from build123d import *

# Parameters (mm, degrees)
ESQUISSE1_R             = 4.415
BOSS_EXTRU_1_DEPTH      = 14.46
ESQUISSE4_R             = 2.9
ENL_V_MAT_EXTRU_1_DEPTH = 14.46
ESQUISSE6_R             = 3.415
ENL_V_MAT_EXTRU_2_DEPTH = 7


with BuildPart() as part:
    # Esquisse1 → Boss.-Extru.1 (new body)
    with BuildSketch(Plane.XY):
        Circle(ESQUISSE1_R)
    extrude(amount=BOSS_EXTRU_1_DEPTH)

    # Esquisse4 → Enlèv. mat.-Extru.1 (cut)
    with BuildSketch(Plane.XY.offset(14.46)):
        Circle(ESQUISSE4_R)
    extrude(amount=-ENL_V_MAT_EXTRU_1_DEPTH, mode=Mode.SUBTRACT)

    # Esquisse6 → Enlèv. mat.-Extru.2 (cut)
    with BuildSketch(Plane.XY.offset(14.46)):
        Circle(ESQUISSE6_R)
    extrude(amount=-ENL_V_MAT_EXTRU_2_DEPTH, mode=Mode.SUBTRACT)


solid = part.part
Could you check a few things on this model? Use its own coordinates, in mm. A direction names the side the tool comes from. Give positions to 0.01 mm unless a question says otherwise; leave off trailing zeros. Order: outer loops, then holes, each group sorted by start corner. A loop starts at its lowest first (then second) coordinate and runs counter-clockwise, first axis right, second up. Notation, with made-up numbers: (49, -37) - (54, -37) arc R18 ccw to (54, -13) - close; hole circle Ø3 at (-3.5, -2.5). An arc over 180 degrees is marked (long way). One line per question, with ' | ' between items. Start each with the question number.
Item 1: I need wall thicknesses on probe 1 along Y at (x, z) = (0, 9.25) (3 decimals); probe 2 along Y at (x, z) = (0, 5.5) (3 decimals); probe 3 along Z at (x, y) = (0.75, 3.25). Which ranges of each line are inside material? Lowest first, please. Write a range as [from, to].
Item 2: I want a section at C-C on z = 3. Write out the boundary of the cut face in (x, y) (3 decimals), then the cut area to 3 significant figures.
Item 3: I want a section at B-B on y = 1. Write out the boundary of the cut face in (x, z), then the cut area to 3 significant figures.
Item 4: I want a section at A-A on x = 0. Write out the boundary of the cut face in (y, z) (3 decimals).
Item 5: I'm going to push a flat-ended pin straight in: pin 1 Ø5 at (x, z) = (-3, 2) entering from +Y. Where does the tip first touch, or does it pass through?
Item 6: For faces 4 (the cylindrical face through (-0.445, 3.386, 11.009)), 5 (the flat face through (2, -3, 14.46)), which set-ups out of +Z, -Z, +X, -X, +Y, -Y let a thin tool reach every point of the face, with its end or its side?
Item 7: Thinking about a two-plate mould opening in X: for faces 1 (the cylindrical face through (-2.9, 0.1, 3.8)), 2 (the flat face through (1, -3, 0)), 3 (the cylindrical face through (-1, -4.3, 7.1)), which applies, pulls with the +X half, pulls with the -X half, needs draft (parallel to the pull), parting line crosses it, or undercut?
Verdict:
1) probe 1: [-4.415, -3.415], [3.415, 4.415] | probe 2: [-4.415, -2.9], [2.9, 4.415] | probe 3: [0, 7.46]
2) outline: circle Ø8.83 at (0, 0); hole circle Ø5.8 at (0, 0) | area: 34.8 mm^2
3) outline: (-4.3, 0) - (-2.72, 0) - (-2.72, 7.46) - (-3.27, 7.46) - (-3.27, 14.46) - (-4.3, 14.46) - close; (2.72, 0) - (4.3, 0) - (4.3, 14.46) - (3.27, 14.46) - (3.27, 7.46) - (2.72, 7.46) - close | area: 38.0 mm^2
4) outline: (-4.415, 0) - (-2.9, 0) - (-2.9, 7.46) - (-3.415, 7.46) - (-3.415, 14.46) - (-4.415, 14.46) - close; (2.9, 0) - (4.415, 0) - (4.415, 14.46) - (3.415, 14.46) - (3.415, 7.46) - (2.9, 7.46) - close
5) pin 1: y = 4.39
6) face 4: +Z | face 5: +Z, +X, -X, +Y, -Y
7) face 1: undercut | face 2: needs draft | face 3: parting line crosses it
